Geometry: final body of the model. Coordinates: model frame, mm. Face numbers are marked on the shaded views. A direction names the side the tool comes from. Coordinates: 2 decimals unless noted, no trailing zeros. Loops run counter-clockwise (first coordinate to the right, second up) from the corner with the lowest first, then second, coordinate; pieces in that order, holes last. Notation, with made-up numbers: (75.25, -35) -> (80.25, -35) arc R23 cw to (80.25, -26) -> close; hole circle Ø6 at (-39.75, -33). An arc over 180 degrees is marked (long way). One line per item, written item: value. Start each with the question number.
Item 1: Section query B-B on z = 0. Return loops of the section in (x, y).
Item 2: Section query C-C on y = 1.1. Return loops of the section in (x, z).
Item 3: Ray query, probe 1 along X at (y, z) = (2.45, 0); probe 2 along Z at (x, y) = (31, 1.9); probe 3 along X at (y, z) = (0.55, -0.75). Return the intervals inside material, ascending. Write a range as from..to.
Item 4: Contact query for flat-ended pins moving along their axis: pin 1 Ø4.5 at (x, z) = (9, 0) entering from +Y; pin 2 Ø2.5 at (x, z) = (-25, 1) entering from +Y. Output: stop coordinate, or through.
Item 5: Section query A-A on x = 31. Return loops of the section in (y, z).
Item 6: Section query D-D on x = -13. Return loops of the section in (y, z), then the cut area to 3 significant figures.
Item 7: Set-up query: the marked faces 1 and 2. Return all of +Z, -Z, +X, -X, +Y, -Y with unobstructed straight access to the full face (end or side cutting, diameter ignored); none if empty.
Autodesk Inventor part; units mm, degrees
ref_plane "YZ Plane" through (0, 0, 0) normal (1, 0, 0) x (0, 1, 0)
ref_plane "XZ Plane" through (0, 0, 0) normal (0, 1, 0) x (-1, 0, 0)
ref_plane "XY Plane" through (0, 0, 0) normal (0, 0, 1) x (1, 0, 0)
sketch "Skizze1" plane through (0, 0, 0) normal (0, 1, 0) x (-1, 0, 0)
  line L0 (-35, 4) -> (35, 4)
  line L1 (35, 4) -> (35, -4)
  line L2 (35, -4) -> (-35, -4)
  line L3 (-35, -4) -> (-35, 4)
  line L4 (-35, 4) -> (35, -4) construction
  line L5 (35, 4) -> (-35, -4) construction
  point P0 (0, 0)
  dimension "d0" = 70
  dimension "d1" = 8
extrude "Extrusion1" add sketch "Skizze1" along normal blind 5
sketch "Skizze2" plane through (0, 5, 0) normal (0, 1, 0) x (1, 0, 0)
  line L0 (-35, -4) -> (35, -4)
  line L1 (35, -4) -> (35, 4)
  line L2 (35, 4) -> (-35, 4)
  line L3 (-35, 4) -> (-35, -4)
  line L4 (0, 0) -> (47.4069, 0) construction
  point P0 (31, 0)
  point P1 (9, 0)
  dimension "d4" = 8
  dimension "d5" = 4
  dimension "d7" = 22
hole "Bohrung1" at (31, 5, 0) at (9, 5, 0) direction (0, -1, 0) diameter 3.4 end through all
sketch "Skizze3" plane through (0, 5, 0) normal (0, 1, 0) x (1, 0, 0)
  line L0 (19.9613, 0) -> (-27.7601, 0) construction
  circle A0 centre (9, 0) radius 1.7
  point P0 (0, 0)
  point P1 (-13, 0)
  point P2 (-28.5, 0)
  dimension "d15" = 22
  dimension "d16" = 15.5
hole "Bohrung2" at (-13, 5, 0) at (-28.5, 5, 0) direction (0, -1, 0) diameter 3.4 end through all
sketch "Skizze4" plane through (0, 5, 0) normal (0, 1, 0) x (1, 0, 0)
  circle A0 centre (-13, 0) radius 1.7
  circle A1 centre (-28.5, 0) radius 1.7
  circle A2 centre (31, 0) radius 1.7
  circle A3 centre (9, 0) radius 1.7
  line L0 (-35, -4) -> (35, -4)
  line L1 (35, -4) -> (35, 4)
  line L2 (35, 4) -> (-35, 4)
  line L3 (-35, 4) -> (-35, -4)
  line L4 (-35, 4) -> (35, 4)
  line L5 (35, -4) -> (4, -4)
  line L6 (4, -4) -> (4, 4)
  line L7 (4, 4) -> (35, 4)
  line L8 (35, 4) -> (35, -4)
  point P0 (0, 0)
  dimension "d27" = 5
extrude "Extrusion2" add sketch "Skizze4" along normal blind 0.5 contours L6 L2 L1 L0
properties part number "connection_hand_camera"
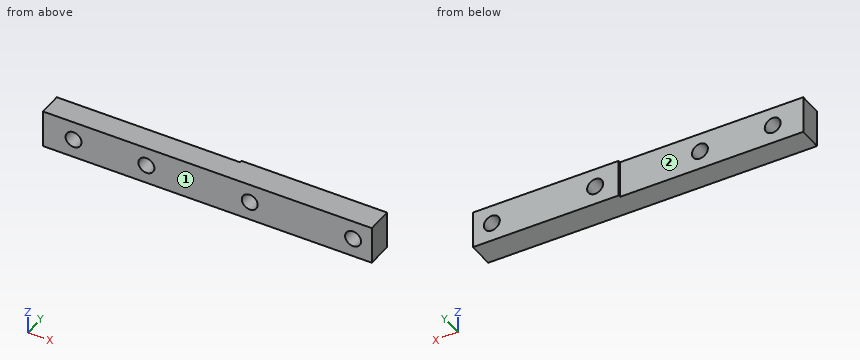
Reply:
1. outline: (-35, 0) -> (-30.2, 0) -> (-30.2, 5) -> (-35, 5) -> close; (-26.8, 0) -> (-14.7, 0) -> (-14.7, 5) -> (-26.8, 5) -> close; (-11.3, 0) -> (7.3, 0) -> (7.3, 5.5) -> (4, 5.5) -> (4, 5) -> (-11.3, 5) -> close; (10.7, 0) -> (29.3, 0) -> (29.3, 5.5) -> (10.7, 5.5) -> close; (32.7, 0) -> (35, 0) -> (35, 5.5) -> (32.7, 5.5) -> close
2. outline: (-35, -4) -> (35, -4) -> (35, 4) -> (-35, 4) -> close; hole circle Ø3.4 at (-28.5, 0); hole circle Ø3.4 at (-13, 0); hole circle Ø3.4 at (9, 0); hole circle Ø3.4 at (31, 0)
3. probe 1: x = -35..-30.2, -26.8..-14.7, -11.3..7.3, 10.7..29.3, 32.7..35
3. probe 2: z = -4..-1.7, 1.7..4
3. probe 3: x = -35..-30.03, -26.97..-14.53, -11.47..7.47, 10.53..29.47, 32.53..35
4. pin 1: stops at y = 5.5
4. pin 2: stops at y = 5
5. outline: (0, -4) -> (5.5, -4) -> (5.5, -1.7) -> (0, -1.7) -> close; (0, 1.7) -> (5.5, 1.7) -> (5.5, 4) -> (0, 4) -> close
6. outline: (0, -4) -> (5, -4) -> (5, -1.7) -> (0, -1.7) -> close; (0, 1.7) -> (5, 1.7) -> (5, 4) -> (0, 4) -> close
6. area: 23.0 mm²
7. face 1: +Z, -Z, +X, -X, -Y
7. face 2: +Z, -Z, -X, +Y
